Here's how the part is built. I have some questions about the finished solid (model axes, mm). Give positions to 0.01 mm unless a question says otherwise; leave off trailing zeros. Order: outer loops, then holes, each group sorted by start corner. A loop starts at its lowest first (then second) coordinate and runs counter-clockwise, first axis right, second up.
Autodesk Inventor part; units mm, degrees
ref_plane "Work Plane1" through (3, 0, 0) normal (0, 0.5, 0.8660254) x (1, 0, 0)
ref_plane "YZ Plane" through (0, 0, 0) normal (1, 0, 0) x (0, 1, 0)
ref_plane "XZ Plane" through (0, 0, 0) normal (0, 1, 0) x (-1, 0, 0)
sketch "Sketch1" plane through (0, 0, 0) normal (0, 0, 1) x (1, 0, 0)
  line L0 (0, 4) -> (0, 0)
  line L1 (0, 0) -> (45, 0)
  line L2 (45, 0) -> (45, 4)
  line L3 (45, 4) -> (0, 4)
  line L4 (-9, 0) -> (54, 0)
  line L5 (0, -0.8) -> (0, 4.8)
  dimension "d0" = 8
  dimension "d1" = 45
revolve "Body" add sketch "Sketch1" angle 360 about axis through (0, 0, 0) along (1, 0, 0)
sketch "Sketch2" plane through (0, 0, 0) normal (1, 0, 0) x (0, 1, 0)
  line L0 (0, 7.5056) -> (6.5, 3.7528)
  line L1 (6.5, 3.7528) -> (6.5, -3.7528)
  line L2 (6.5, -3.7528) -> (0, -7.5056)
  line L3 (0, -7.5056) -> (-6.5, -3.7528)
  line L4 (-6.5, -3.7528) -> (-6.5, 3.7528)
  line L5 (-6.5, 3.7528) -> (0, 7.5056)
  line L6 (-9.1, 0) -> (9.1, 0)
  line L7 (0, -10.5078) -> (0, 10.5078)
  point P0 (0, 0)
  point P1 (0, 0)
  dimension "d2" = 13
extrude "Head" add sketch "Sketch2" against normal blind 6.5
sketch "Sketch3" plane through (-6.5, 0, 0) normal (-1, 0, 0) x (0, 1, 0)
  circle A0 centre (0, 0) radius 4.875
  point P0 (0, 0)
  dimension "d12" = 9.75
extrude "Indent1" cut sketch "Sketch3" against normal blind 1.3
sketch "Sketch4" plane through (0, 0, 0) normal (0, 0, 1) x (1, 0, 0)
  line L0 (-6.5, 7.5056) -> (-6.5, 6.5)
  line L1 (-6.5, 6.5) -> (-5.9194, 7.5056)
  line L2 (-5.9194, 7.5056) -> (-6.5, 7.5056)
  line L3 (0, 7.5056) -> (0, 6.5)
  line L4 (0, 6.5) -> (-0.5806, 7.5056)
  line L5 (-0.5806, 7.5056) -> (0, 7.5056)
  line L6 (0, 0) -> (-6.5, 0)
  line L7 (-6.5, 0) -> (-6.5, 6.5)
  line L8 (0, 0) -> (0, 6.5)
  line L9 (-7.8, 0) -> (1.3, 0)
  line L10 (-5.9194, 7.5056) -> (-0.5806, 7.5056) construction
  line L11 (0, -1.5011) -> (0, 9.0067)
  dimension "d6" = 30
  dimension "d7" = 30
  dimension "d16" = 13
  dimension "d17" = 13
  dimension "d18" = 15.0111
revolve "Chamfer1" cut sketch "Sketch4" angle 360 about axis through (-10, 0, 0) along (1, 0, 0)
fillet "Fillet1" radius 0.4 1 edges at (0, -4, 0)
thread "Thread"
ref_plane "Work Plane1" through (3, 0, 0) normal (0, 0.5, 0.8660254) x (1, 0, 0)
equation "\"d2\" = SW"
equation "\"d3\" = KOH"
equation "\"d12\" = 0.75 * SW0"
equation "\"d14\" = 0.2 * KOH"
equation "\"d11\" = RR"
equation "\"d8\" = GEL"
equation "\"d0\" = GD"
equation "\"d1\" = NLG"
equation "\"d6\" = ANG1"
equation "\"d7\" = ANG1"
equation "\"d16\" = SW0"
equation "\"d17\" = SW0"
equation "\"d18\" = 1.1547 * SW"
equation "\"NLG\" = 45"
equation "\"KOH\" = 6.5"
equation "\"GD\" = NND"
equation "\"GEL\" = 42.5"
equation "\"SW\" = 13"
equation "\"SW0\" = SW"
equation "\"ANG1\" = 30deg"
equation "\"RR\" = 0.4"
equation "\"GUL\" = 0.61345 * PTC"
equation "\"SPD\" = NND - 1.2269 * PTC"
equation "\"GD1\" = THREADDIA - 1.2269 * PTC"
equation "\"THREADDIA\" = 8"
equation "\"SDH\" = 9.2"
equation "\"TOA\" = 30deg"
equation "\"BDM\" = NND"
equation "\"FAWI\" = 45deg"
equation "\"PTC\" = 1.25"
equation "\"NND\" = 8"
equation "\"GAL\" = 0.61345 * PTC"
equation "\"SD\" = 0"
equation "\"SD2\" = SDH"
equation "\"E0\" = 1.155 * SW"
properties part number "AS 1427 - M8 x 45" material "Steel, Mild"
Q1. I need wall thicknesses on L1, parallel to Y at x = -5.5, z = 0 (3 decimals); L2, parallel to X at y = 3.75, z = -4.25; L3, parallel to Z at x = -5.95, y = 0 (3 decimals). Which ranges of each line are inside material? Lowest first, please.
Filled sheet:
L1: y = -6.5 to -4.875, 4.875 to 6.5
L2: x = -6.5 to 0
L3: z = -7.453 to -4.875, 4.875 to 7.453
Q2. I'm going to push flat-ended pins straight in: P1, Ø1, axis at y = 3.5, z = -0.5, coming from the -X side; P2, Ø1.5, axis at y = 5, z = -1, coming from the +X side; P3, Ø6, axis at x = 13, z = -6, coming from the -Y side. Where does each tip first touch, or does it pass through?
Filled sheet:
P1: stops at x = -5.2
P2: stops at x = 0
P3: stops at y = -2.65
Q3. If we section it at A-A on x = 19: List the corners of the cut face in (y, z) for me, plus the area to 3 significant figures.
Filled sheet:
outline: circle Ø8 at (0, 0)
area: 50.3 mm2
Q4. Thinking about a two-plate mould opening in Z: for faces 1 (the face through (-0.12, 0.02, -6.71)), 2 (the face through (-5.859, -0.635, -4.834)), 3 (the face through (22.388, -0.867, 3.905)), 4 (the face through (-3.2, -3.3, 5.6)), which applies, released by +Z, released by -Z, zero draft, split by the parting line, or undercut?
Filled sheet:
face 1: released by -Z
face 2: undercut
face 3: split by the parting line
face 4: released by +Z
